Here's the drawing with two shaded views (mm, measured from the low corner). I have some questions. A direction names the side the tool comes from. Give positions to 0.01 mm unless a question says otherwise; leave off trailing zeros. Write each loop counter-clockwise with the first axis right and the second up, starting at its lowest first coordinate (ties: lowest second). Pieces come first, ordered by that corner, then holes.
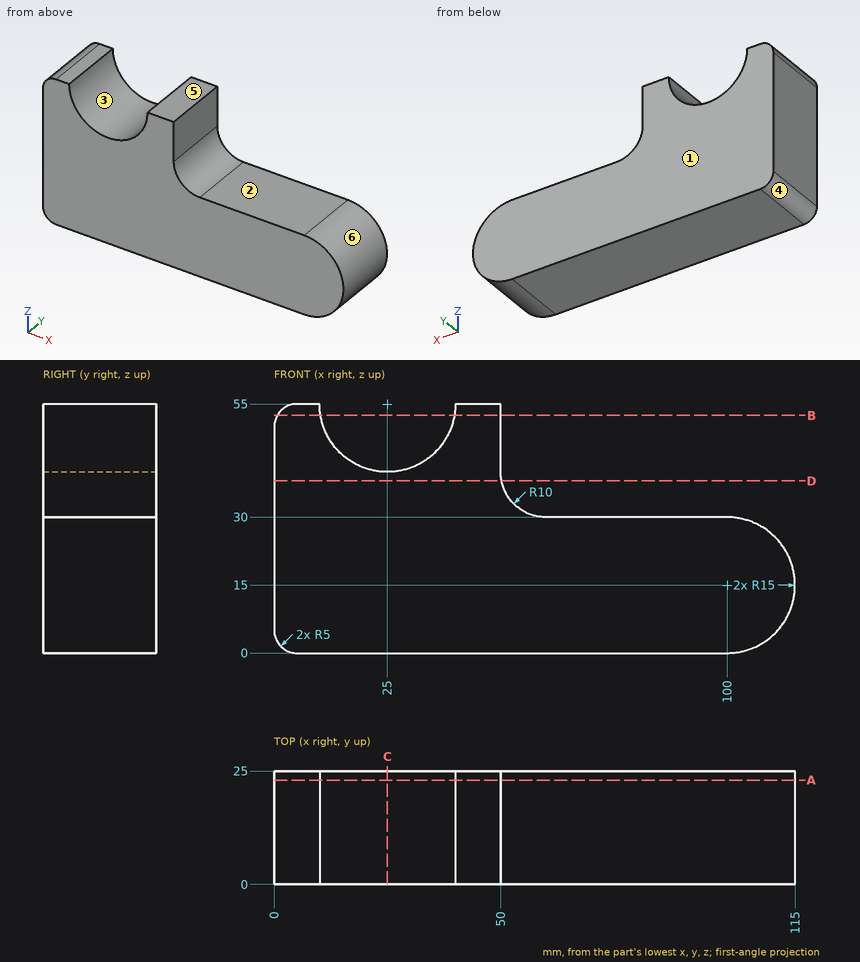
1) If we mould it in two halves opening along X, with no side actions, what happens to the marked faces 3, 4, 5 and 6? For each: +X half, -X half, draft (parallel to the pull), parting line (faces both ways), or undercut.
Values follow:
face 3: undercut
face 4: -X half
face 5: draft
face 6: +X half
2) Suppose I cut it at B-B on z = 52.5. Write out the boundary of the cut face in (x, y), plus the area to 3 significant figures.
Values follow:
outline: (0.67, 0) - (10.21, 0) - (10.21, 25) - (0.67, 25) - close; (39.79, 0) - (50, 0) - (50, 25) - (39.79, 25) - close
area: 494 mm2
3) Suppose I cut it at D-D on z = 38. Write out the boundary of the cut face in (x, y), plus the area to 3 significant figures.
Values follow:
outline: (0, 0) - (50.2, 0) - (50.2, 25) - (0, 25) - close
area: 1,260 mm2
4) For the marked faces 1 and 2, which set-ups out of +Z, -Z, +X, -X, +Y, -Y let a thin tool reach every point of the face, with its end or its side?
Values follow:
face 1: +Z, -Z, +X, -X, +Y
face 2: +Z, +X, +Y, -Y
5) For pin 1 Ø3 at (y, z) = (20.5, 46.5) entering from +X; pin 2 Ø3 at (y, z) = (3.5, 17.5) entering from +X; pin 3 Ø1 at (y, z) = (3, 29) entering from +X, each with a flat end and sliding along its axis, tell me the tip position at first contact or that it passes through.
Values follow:
pin 1: stops at x = 50
pin 2: stops at x = 114.97
pin 3: stops at x = 106.54
6) Suppose I cut it at C-C on x = 25. Write out the boundary of the cut face in (y, z), plus the area to 3 significant figures.
Values follow:
outline: (0, 0) - (25, 0) - (25, 40) - (0, 40) - close
area: 1,000 mm2
7) Suppose I cut it at A-A on y = 23. Write out the boundary of the cut face in (x, z), plus the area to 3 significant figures.
Values follow:
outline: (0, 5) arc R5 ccw to (5, 0) - (100, 0) arc R15 ccw to (100, 30) - (60, 30) arc R10 cw to (50, 40) - (50, 55) - (40, 55) arc R15 cw to (10, 55) - (5, 55) arc R5 ccw to (0, 50) - close
area: 4,260 mm2
8) Please list where these lines run through material, in increasing order: L1, parallel to X at y = 17, z = 42; L2, parallel to X at y = 5.25, z = 51.5; L3, parallel to Z at x = 75.5, y = 10.25.
Values follow:
L1: x = 0 to 17.52, 32.48 to 50
L2: x = 0.23 to 10.41, 39.59 to 50
L3: z = 0 to 30
